from build123d import *

# Parameters (mm, degrees)
SKETCH1_R                = 42.9
BOSS_EXTRUDE1_DEPTH      = 2.5
BOSS_EXTRUDE1_DEPTH_BACK = 30.3
CHAMFER1_SIZE            = 10
CHAMFER1_SIZE2           = 17.320508076
FILLET1_R                = 6
SHELL1_T                 = -2.4
CUT_EXTRUDE1_REACH       = 83.441
SKETCH2_R                = 3.925
SKETCH2_R_2              = 1.375
SKETCH3_R                = 2.675
CUT_EXTRUDE2_DEPTH       = 1.4


with BuildPart() as part:
    # Sketch1 → Boss-Extrude1 (new, two sides)
    with BuildSketch(Plane.XY) as boss_extrude1_sk:
        with Locations(Location((9.62, 10, 0), (0, 0, 90))):
            Circle(SKETCH1_R)
    extrude(amount=BOSS_EXTRUDE1_DEPTH)
    extrude(boss_extrude1_sk.sketch, amount=-BOSS_EXTRUDE1_DEPTH_BACK)

    # Chamfer1
    chamfer1_edges = [part.edges().sort_by_distance(p)[0] for p in [
        (9.62, -32.9, 2.5),
    ]]
    chamfer1_side = [part.faces().sort_by_distance(p)[0] for p in [
        (9.62, 10, 2.5),
    ]]
    chamfer(chamfer1_edges, length=CHAMFER1_SIZE, length2=CHAMFER1_SIZE2, reference=chamfer1_side[0])

    # Fillet1
    fillet1_edges = [part.edges().sort_by_distance(p)[0] for p in [
        (9.62, -32.9, -14.820508076),
    ]]
    fillet(fillet1_edges, radius=FILLET1_R)

    # Shell1
    shell1_openings = [part.faces().sort_by_distance(p)[0] for p in [
        (9.62, 10, -30.3),
    ]]
    offset(amount=SHELL1_T, openings=shell1_openings, kind=Kind.INTERSECTION)

    # Sketch2 → Cut-Extrude1 (cut, up to next)
    with BuildSketch(Plane.XY.offset(2.5), mode=Mode.PRIVATE) as cut_extrude1_sk1:
        with Locations((9.62, 10)):
            Circle(SKETCH2_R)
    cut_extrude1_tool1 = extrude(cut_extrude1_sk1.sketch, amount=-CUT_EXTRUDE1_REACH, mode=Mode.PRIVATE) & part.part
    # Sketch2 → Cut-Extrude1 (cut, up to next)
    with BuildSketch(Plane.XY.offset(2.5), mode=Mode.PRIVATE) as cut_extrude1_sk2:
        with Locations((9.62, 17.285)):
            Circle(SKETCH2_R_2)
    cut_extrude1_tool2 = extrude(cut_extrude1_sk2.sketch, amount=-CUT_EXTRUDE1_REACH, mode=Mode.PRIVATE) & part.part
    # Sketch2 → Cut-Extrude1 (cut, up to next)
    with BuildSketch(Plane.XY.offset(2.5), mode=Mode.PRIVATE) as cut_extrude1_sk3:
        with Locations((9.62, 2.715)):
            Circle(SKETCH2_R_2)
    cut_extrude1_tool3 = extrude(cut_extrude1_sk3.sketch, amount=-CUT_EXTRUDE1_REACH, mode=Mode.PRIVATE) & part.part
    # Sketch2 → Cut-Extrude1 (cut, up to next)
    with BuildSketch(Plane.XY.offset(2.5), mode=Mode.PRIVATE) as cut_extrude1_sk4:
        with Locations((2.335, 10)):
            Circle(SKETCH2_R_2)
    cut_extrude1_tool4 = extrude(cut_extrude1_sk4.sketch, amount=-CUT_EXTRUDE1_REACH, mode=Mode.PRIVATE) & part.part
    # Sketch2 → Cut-Extrude1 (cut, up to next)
    with BuildSketch(Plane.XY.offset(2.5), mode=Mode.PRIVATE) as cut_extrude1_sk5:
        with Locations((16.905, 10)):
            Circle(SKETCH2_R_2)
    cut_extrude1_tool5 = extrude(cut_extrude1_sk5.sketch, amount=-CUT_EXTRUDE1_REACH, mode=Mode.PRIVATE) & part.part
    add(cut_extrude1_tool1.solids().sort_by_distance((9.62, 10, 2.5))[0], mode=Mode.SUBTRACT)
    add(cut_extrude1_tool2.solids().sort_by_distance((9.62, 17.285, 2.5))[0], mode=Mode.SUBTRACT)
    add(cut_extrude1_tool3.solids().sort_by_distance((9.62, 2.715, 2.5))[0], mode=Mode.SUBTRACT)
    add(cut_extrude1_tool4.solids().sort_by_distance((2.335, 10, 2.5))[0], mode=Mode.SUBTRACT)
    add(cut_extrude1_tool5.solids().sort_by_distance((16.905, 10, 2.5))[0], mode=Mode.SUBTRACT)

    # Sketch3 → Cut-Extrude2 (cut)
    with BuildSketch(Plane.XY.offset(2.5)):
        with Locations((2.335, 10)):
            Circle(SKETCH3_R)
        with Locations((9.62, 2.715)):
            Circle(SKETCH3_R)
        with Locations((9.62, 17.285)):
            Circle(SKETCH3_R)
        with Locations((16.905, 10)):
            Circle(SKETCH3_R)
    extrude(amount=-CUT_EXTRUDE2_DEPTH, mode=Mode.SUBTRACT)


solid = part.part
Source: CAD feature listing. Evaluate the final solid. Frame: model axes, mm. A direction names the side the tool comes from. Coordinates: 2 decimals unless noted, no trailing zeros. Loops run counter-clockwise (first coordinate to the right, second up) from the corner with the lowest first, then second, coordinate; pieces in that order, holes last. Notation, with made-up numbers: (35, 59.25) - (54, 59.25) arc R20 cw to (54, 90.25) - close; hole circle Ø11 at (77.5, 79). An arc over 180 degrees is marked (long way). One line per question, with ' | ' between items.
1) First-contact query: P1, Ø4.5, axis at x = 16.905, y = 10, coming from the +Z side; P2, Ø12, axis at x = -6.5, z = -23, coming from the +Y side; P3, Ø8, axis at x = -18, z = -19, coming from the +Y side; P4, Ø6, axis at x = 11, y = 16, coming from the +Z side. Flat tips, straight axial feed; report the tip coordinate or a pass-through.
Report:
P1: stops at z = 1.1 | P2: stops at y = 51.69 | P3: stops at y = 45.81 | P4: stops at z = 2.5
2) Section A-A, the plane x = 9.62. Give the number of separate pieces and of enclosed holes in the cut face, then the cut area to 3 significant figures.
Report:
separate pieces: 4 | enclosed holes: 0 | area: 279 mm²
3) Line query: line 1 along Z through (x, y) = (1, -6.5); line 2 along X through (y, z) = (10, -22); line 3 along X through (y, z) = (21.5, -17.5). Output: solid intervals per line, ascending.
Report:
line 1: z = 0.1 to 2.5 | line 2: x = -33.28 to -30.88, 50.12 to 52.52 | line 3: x = -31.71 to -29.21, 48.45 to 50.95
4) Set-up query: faces 1 (the face through (8.77, 6.17, 1.32)), 2 (the face through (6.948, 2.833, 1.81)), 3 (the face through (16, 17, 0.1)). Return all of +Z, -Z, +X, -X, +Y, -Y with unobstructed straight access to the full face (end or side cutting, diameter ignored); none if empty.
Report:
face 1: +Z, -Z | face 2: +Z | face 3: -Z
5) Section D-D, the plane z = -1.5. Return loops of the section in (x, y), then the cut area to 3 significant figures.
Report:
outline: circle Ø70.42 at (9.62, 10); hole circle Ø64.88 at (9.62, 10) | area: 589 mm²
6) Section C-C, the plane z = -27.5. Return loops of the section in (x, y), then the cut area to 3 significant figures.
Report:
outline: circle Ø85.8 at (9.62, 10); hole circle Ø81 at (9.62, 10) | area: 629 mm²
